The figure shows three views and two pictorial views of one solid part (mm, origin at its lowest corner). Answer the questions. Round coordinates to 2 decimals unless told otherwise and drop trailing zeros. Write each loop counter-clockwise with the first axis right and the second up, starting at its lowest first coordinate (ties: lowest second). Pieces come first, ordered by that corner, then holes. Notation, with made-up numbers: M 77,16 L 110,16 A28 cw 110,50 Z; hole C 7,-6.75 d2. An arc over 180 degrees is marked long. One line per item, written item: value. Start each with the question number.
Q1. Find section A-A (z = 15). Write down the section's boundary in (x, y).
Q2. Find section D-D (z = 22.5). Write down the section's boundary in (x, y).
Q3. Find section B-B (x = 35). Write down the section's boundary in (y, z), and give its area (3 significant figures).
Q4. Find section C-C (z = 10). Write down the section's boundary in (x, y), and give its area (3 significant figures).
Q5. Given pin 1 Ø0.5 at (x, y) = (5.5, 1) entering from -Z; pin 2 Ø0.5 at (y, z) = (0.5, 27.5) entering from +X; pin 3 Ø0.5 at (x, y) = (72, 0.5) entering from +Z, each flat-ended and moving along its own axis, determine where each tip first touches the part or whether it passes through.
Q6. Consider probe 1 along X at (y, z) = (0.45, 15.5); probe 2 along Z at (x, y) = (55.5, 0.15); probe 3 along X at (y, z) = (0.75, 9). Determine where each line is inside the solid, lowest interval first.
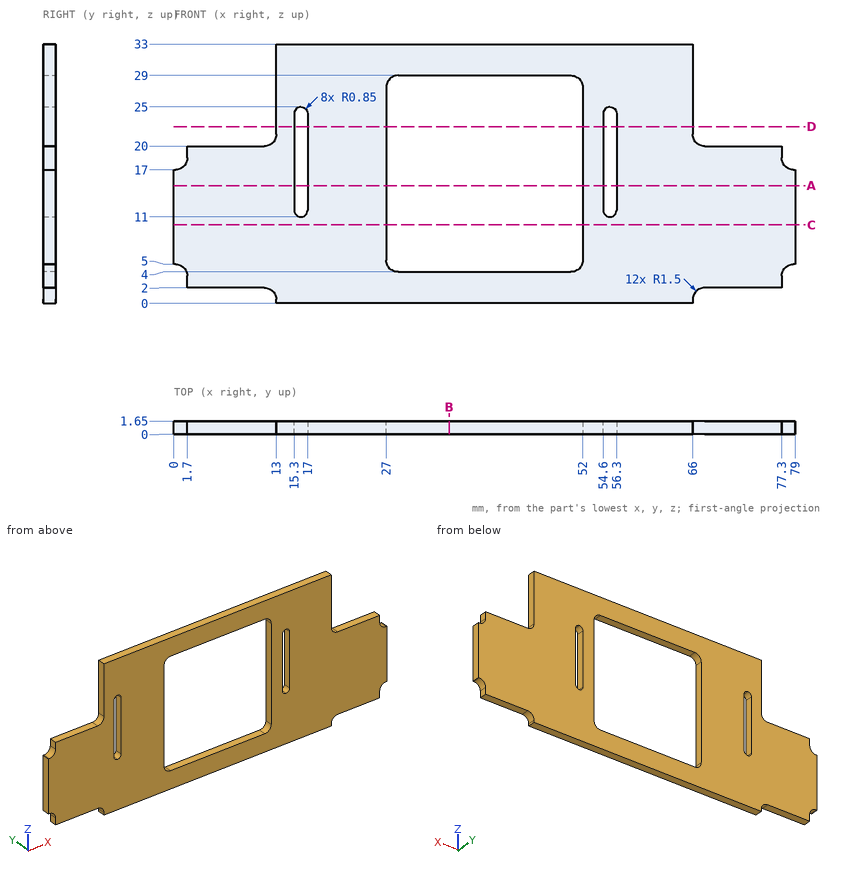
The answers:
1. outline: M 0,0 L 15.3,0 L 15.3,1.65 L 0,1.65 Z; M 17,0 L 27,0 L 27,1.65 L 17,1.65 Z; M 52,0 L 54.6,0 L 54.6,1.65 L 52,1.65 Z; M 56.3,0 L 79,0 L 79,1.65 L 56.3,1.65 Z
2. outline: M 13,0 L 15.3,0 L 15.3,1.65 L 13,1.65 Z; M 17,0 L 27,0 L 27,1.65 L 17,1.65 Z; M 52,0 L 54.6,0 L 54.6,1.65 L 52,1.65 Z; M 56.3,0 L 66,0 L 66,1.65 L 56.3,1.65 Z
3. outline: M 0,0 L 1.65,0 L 1.65,4 L 0,4 Z; M 0,29 L 1.65,29 L 1.65,33 L 0,33 Z
3. area: 13.2 mm2
4. outline: M 0,0 L 27,0 L 27,1.65 L 0,1.65 Z; M 52,0 L 79,0 L 79,1.65 L 52,1.65 Z
4. area: 89.1 mm2
5. pin 1: z = 2
5. pin 2: x = 66
5. pin 3: z = 20
6. probe 1: 0 to 15.3, 17 to 27, 52 to 54.6, 56.3 to 79
6. probe 2: 0 to 11, 25 to 33
6. probe 3: 0 to 27, 52 to 79
